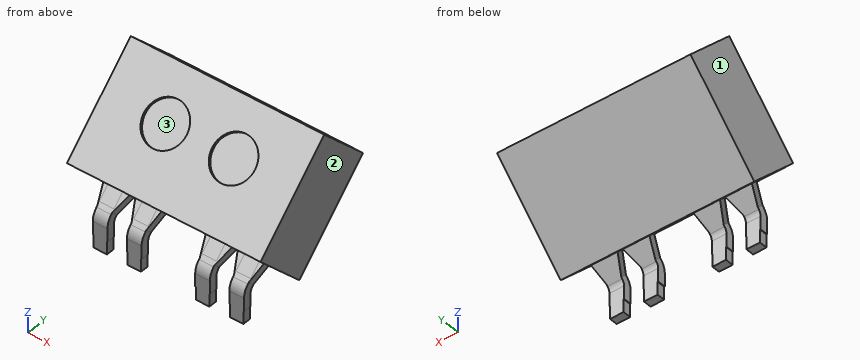
```python
from build123d import *

# Parameters (mm, degrees)
ESQUISSE2_W          = 7.2
ESQUISSE2_H          = 2.5
BOITIER_DEPTH        = 4.1
FENETRECAPTEUR_START = -1.45
ESQUISSE4_R          = 0.8
FENETRECAPTEUR_DEPTH = 0.1
PATTES_DEPTH         = 0.15
PLIAGE_START         = -5
PLIAGE_1_OUTLINE_W   = 7.2
PLIAGE_1_OUTLINE_H   = 4.1
PLIAGE_1_DEPTH       = 4.301040764
PLIAGE_START_2       = -0.698959236
PLIAGE_1_2_OUTLINE_R = 0.8
PLIAGE_1_2_DEPTH     = 0.1
PLIAGE_START_3       = -0.598959236
PLIAGE_1_3_OUTLINE_W = 7.2
PLIAGE_1_3_OUTLINE_H = 4.1
PLIAGE_1_3_DEPTH     = 2.4
PLIAGE_1_4_OUTLINE_W = 7.2
PLIAGE_1_4_OUTLINE_H = 4.1
PLIAGE_1_4_OUTLINE_R = 0.8
PLIAGE_1_4_DEPTH     = 0.1
PLIAGE_START_4       = -3.6
PLIAGE_1_5_DEPTH     = 7.2
PLIAGE_START_5       = -2.813242849
PLIAGE_1_6_DEPTH     = 0.546485698
PLIAGE_START_6       = -1.543242849
PLIAGE_1_7_DEPTH     = 0.546485698
PLIAGE_START_7       = 0.996757151
PLIAGE_1_8_DEPTH     = 0.546485698
PLIAGE_START_8       = 2.266757151
PLIAGE_1_9_DEPTH     = 0.546485698
PLIAGE_START_9       = 0.601040763
PLIAGE_1_10_DEPTH    = 0.300000001


with BuildPart() as part:
    # Esquisse2 → Boitier (new body)
    with BuildSketch(Plane.XY):
        with Locations((0, -0.2)):
            Rectangle(ESQUISSE2_W, ESQUISSE2_H)
    extrude(amount=BOITIER_DEPTH)

    # Esquisse4 → FenetreCapteur (cut)
    with BuildSketch(Plane(origin=(0, 0, 0), x_dir=(1, 0, 0), z_dir=(0, 1, 0)).offset(FENETRECAPTEUR_START)):
        with Locations(Location((-1.27, -2.3, 0), (0, 0, 180))):
            Circle(ESQUISSE4_R)
        with Locations(Location((1.27, -2.3, 0), (0, 0, 180))):
            Circle(ESQUISSE4_R)
    extrude(amount=FENETRECAPTEUR_DEPTH, mode=Mode.SUBTRACT)

    # Esquisse5 → Pattes (add, symmetric)
    with BuildSketch(Plane(origin=(0, 0, 0), x_dir=(1, 0, 0), z_dir=(0, 1, 0))):
        Polygon((2.791437744, 2.2), (2.283797649, 2.2), (2.283797649, 1.724539267), (2.266757151, 1.724539267), (2.266757151, 0.7), (2.002499851, 0), (2.991852509, 0), (2.813242849, 0.7), (2.813242849, 1.724539267), (2.791437744, 1.724539267), align=None)
        Polygon((1.526202351, 2.2), (1.018562256, 2.2), (1.018562256, 1.724539267), (0.996757151, 1.724539267), (0.996757151, 0.7), (0.818147491, 0), (1.807500149, 0), (1.543242849, 0.7), (1.543242849, 1.724539267), (1.526202351, 1.724539267), align=None)
        Polygon((-1.018562256, 2.2), (-1.526202351, 2.2), (-1.526202351, 1.724539267), (-1.543242849, 1.724539267), (-1.543242849, 0.7), (-1.807500149, 0), (-0.818147491, 0), (-0.996757151, 0.7), (-0.996757151, 1.724539267), (-1.018562256, 1.724539267), align=None)
        Polygon((-2.283797649, 2.2), (-2.791437744, 2.2), (-2.791437744, 1.724539267), (-2.813242849, 1.724539267), (-2.813242849, 0.7), (-2.991852509, 0), (-2.002499851, 0), (-2.266757151, 0.7), (-2.266757151, 1.724539267), (-2.283797649, 1.724539267), align=None)
    extrude(amount=PATTES_DEPTH, both=True)

    # Pliage 1: read off the stored shape, not the designer's step
    # Pliage 1 outline → Pliage 1 (cut)
    with BuildSketch(Plane(origin=(0, 0, 0), x_dir=(1, 0, 0), z_dir=(0, 0.707106781186546, -0.707106781186549)).offset(PLIAGE_START)):
        with Locations((0, -2.236827202)):
            Rectangle(PLIAGE_1_OUTLINE_W, PLIAGE_1_OUTLINE_H)
    extrude(amount=PLIAGE_1_DEPTH, mode=Mode.SUBTRACT)

    # Pliage 1 2 outline → Pliage 1 2 (cut)
    with BuildSketch(Plane(origin=(0, 0, 0), x_dir=(1, 0, 0), z_dir=(0, 0.707106781186546, -0.707106781186549)).offset(PLIAGE_START_2)):
        with Locations((-1.27, -2.486827202)):
            Circle(PLIAGE_1_2_OUTLINE_R)
        with Locations((1.27, -2.486827202)):
            Circle(PLIAGE_1_2_OUTLINE_R)
    extrude(amount=PLIAGE_1_2_DEPTH, mode=Mode.SUBTRACT)

    # Pliage 1 3 outline → Pliage 1 3 (add)
    with BuildSketch(Plane(origin=(0, 0, 0), x_dir=(1, 0, 0), z_dir=(0, 0.707106781186546, -0.707106781186549)).offset(PLIAGE_START_3)):
        with Locations((0, -2.236827202)):
            Rectangle(PLIAGE_1_3_OUTLINE_W, PLIAGE_1_3_OUTLINE_H)
    extrude(amount=PLIAGE_1_3_DEPTH)

    # Pliage 1 4 outline → Pliage 1 4 (add)
    with BuildSketch(Plane(origin=(0, 0, 0), x_dir=(1, 0, 0), z_dir=(0, 0.707106781186546, -0.707106781186549)).offset(PLIAGE_START_2)):
        with Locations((0, -2.236827202)):
            Rectangle(PLIAGE_1_4_OUTLINE_W, PLIAGE_1_4_OUTLINE_H)
        with Locations((-1.27, -2.486827202)):
            Circle(PLIAGE_1_4_OUTLINE_R, mode=Mode.SUBTRACT)
        with Locations((1.27, -2.486827202)):
            Circle(PLIAGE_1_4_OUTLINE_R, mode=Mode.SUBTRACT)
    extrude(amount=PLIAGE_1_4_DEPTH)

    # Pliage 1 5 outline → Pliage 1 5 (cut)
    with BuildSketch(Plane.YZ.offset(PLIAGE_START_4)):
        with BuildLine():
            Line((0.021781873, -0.828218127), (0.15, -0.7))
            Line((0.15, -0.7), (0.15, 0))
            Line((0.15, 0), (0.264213563, 0))
            Line((0.264213563, 0), (-1.35, 1.614213563))
            Line((-1.35, 1.614213563), (-1.45, 1.714213563))
            Line((-1.45, 1.714213563), (-1.45, 0))
            Line((-1.45, 0), (-0.15, 0))
            Line((-0.15, 0), (-0.15, -1.242936254))
            ThreePointArc((-0.15, -1.242936254), (-0.105355346, -1.018492421), (0.021781873, -0.828218127))
        make_face()
    extrude(amount=PLIAGE_1_5_DEPTH, mode=Mode.SUBTRACT)

    # Pliage 1 6 outline → Pliage 1 6 (add)
    with BuildSketch(Plane.YZ.offset(PLIAGE_START_5)):
        with BuildLine():
            Line((0.769238816, -0.505025253), (0.557106781, -0.292893218))
            Line((0.557106781, -0.292893218), (0.15, -0.7))
            Line((0.15, -0.7), (0.15, -1.242936254))
            ThreePointArc((0.15, -1.242936254), (0.171808514, -1.133297451), (0.233913907, -1.040350162))
            Line((0.233913907, -1.040350162), (0.769238816, -0.505025253))
        make_face()
    extrude(amount=PLIAGE_1_6_DEPTH)

    # Pliage 1 7 outline → Pliage 1 7 (add)
    with BuildSketch(Plane.YZ.offset(PLIAGE_START_6)):
        with BuildLine():
            Line((0.769238816, -0.505025253), (0.557106781, -0.292893218))
            Line((0.557106781, -0.292893218), (0.15, -0.7))
            Line((0.15, -0.7), (0.15, -1.242936254))
            ThreePointArc((0.15, -1.242936254), (0.171808514, -1.133297451), (0.233913907, -1.040350162))
            Line((0.233913907, -1.040350162), (0.769238816, -0.505025253))
        make_face()
    extrude(amount=PLIAGE_1_7_DEPTH)

    # Pliage 1 8 outline → Pliage 1 8 (add)
    with BuildSketch(Plane.YZ.offset(PLIAGE_START_7)):
        with BuildLine():
            Line((0.769238816, -0.505025253), (0.557106781, -0.292893218))
            Line((0.557106781, -0.292893218), (0.15, -0.7))
            Line((0.15, -0.7), (0.15, -1.242936254))
            ThreePointArc((0.15, -1.242936254), (0.171808514, -1.133297451), (0.233913907, -1.040350162))
            Line((0.233913907, -1.040350162), (0.769238816, -0.505025253))
        make_face()
    extrude(amount=PLIAGE_1_8_DEPTH)

    # Pliage 1 9 outline → Pliage 1 9 (add)
    with BuildSketch(Plane.YZ.offset(PLIAGE_START_8)):
        with BuildLine():
            Line((0.769238816, -0.505025253), (0.557106781, -0.292893218))
            Line((0.557106781, -0.292893218), (0.15, -0.7))
            Line((0.15, -0.7), (0.15, -1.242936254))
            ThreePointArc((0.15, -1.242936254), (0.171808514, -1.133297451), (0.233913907, -1.040350162))
            Line((0.233913907, -1.040350162), (0.769238816, -0.505025253))
        make_face()
    extrude(amount=PLIAGE_1_9_DEPTH)

    # Pliage 1 10 outline → Pliage 1 10 (add)
    with BuildSketch(Plane(origin=(0, 0, 0), x_dir=(1, 0, 0), z_dir=(0, 0.707106781186546, -0.707106781186549)).offset(PLIAGE_START_9)):
        Polygon((2.813242849, 0.513172798), (2.813242849, -0.186827202), (2.991852509, -0.186827202), align=None)
        Polygon((-2.991852509, -0.186827202), (-2.813242849, -0.186827202), (-2.813242849, 0.513172798), align=None)
        Polygon((-2.266757151, -0.186827202), (-2.002499851, -0.186827202), (-2.266757151, 0.513172798), align=None)
        Polygon((-1.807500149, -0.186827202), (-1.543242849, -0.186827202), (-1.543242849, 0.513172798), align=None)
        Polygon((-0.996757151, -0.186827202), (-0.818147491, -0.186827202), (-0.996757151, 0.513172798), align=None)
        Polygon((0.818147491, -0.186827202), (0.996757151, -0.186827202), (0.996757151, 0.513172798), align=None)
        Polygon((1.543242849, -0.186827202), (1.807500149, -0.186827202), (1.543242849, 0.513172798), align=None)
        Polygon((2.266757151, 0.513172798), (2.002499851, -0.186827202), (2.266757151, -0.186827202), align=None)
    extrude(amount=PLIAGE_1_10_DEPTH)


solid = part.part
```
Design review of the part built by this model. Coordinates are the model's own, in mm. Face numbers are marked on the shaded views. Coordinates: 2 decimals unless noted, no trailing zeros. Write each loop counter-clockwise with the first axis right and the second up, starting at its lowest first coordinate (ties: lowest second). Pieces come first, ordered by that corner, then holes.
1) Add section A-A (z = -1.55). Write out the cut boundary in (x, y), plus the area to 3 significant figures.
2) Mouldability with a two-part tool opening along X and no side actions: class the marked faces 1, 2 and 3 as +X half, -X half, draft (parallel to the pull), parting line (faces both ways), or undercut.
3) Insertion check: pin 1 (0.5 mm diameter, centred on y = 0, z = -1, fed in from +X); pin 2 (3 mm diameter, centred on x = -1.5, z = 1.5, fed in from +Y); pin 3 (1.5 mm diameter, centred on x = 0, y = 0.5, fed in from +Z); pin 4 (0.5 mm diameter, centred on y = 0, z = -1, fed in from -X). Each pin has a flat end and moves straight along its axis. Give the tip position at first contact, or say it passes through.
4) Add section C-C (x = 2.5). Write out the cut boundary in (y, z).
5) Add section D-D (y = 2.1). Write out the cut boundary in (x, z), plus the area to 3 significant figures.
6) Add section B-B (y = 0.45). Write out the cut boundary in (x, z), plus the area to 4 significant figures.
7) To check wall thickness, follow L1, parallel to Z at x = 0, y = 0; L2, parallel to Y at x = 0, z = 1.25; L3, parallel to Z at x = -1.5, y = -0.2. State the ranges of each line that lie inside material, in increasing order.
Check result:
1. outline: (-2.81, -0.15) - (-2.27, -0.15) - (-2.27, 0.15) - (-2.81, 0.15) - close; (-1.54, -0.15) - (-1, -0.15) - (-1, 0.15) - (-1.54, 0.15) - close; (1, -0.15) - (1.54, -0.15) - (1.54, 0.15) - (1, 0.15) - close; (2.27, -0.15) - (2.81, -0.15) - (2.81, 0.15) - (2.27, 0.15) - close
1. area: 0.656 mm2
2. face 1: -X half
2. face 2: +X half
2. face 3: undercut
3. pin 1: stops at x = 2.83
3. pin 2: stops at y = 4.3
3. pin 3: stops at z = 2.24
3. pin 4: stops at x = -2.83
4. outline: (-0.36, 0.63) - (0.56, -0.29) - (0.02, -0.83) arc R0.59 ccw to (-0.15, -1.24) - (-0.15, -2.2) - (0.15, -2.2) - (0.15, -1.24) arc R0.29 cw to (0.23, -1.04) - (0.77, -0.51) - (1.41, -1.14) - (4.3, 1.76) - (2.54, 3.53) - close
5. outline: (-3.6, -0.45) - (3.6, -0.45) - (3.6, 3.09) - (-3.6, 3.09) - close
5. area: 25.5 mm2
6. outline: (-3.6, -0.19) - (3.6, -0.19) - (3.6, 1.44) - (-3.6, 1.44) - close; (-2.95, -0.4) - (-2.88, -0.82) - (-2.17, -0.82) - (-2.06, -0.4) - close; (-1.75, -0.4) - (-1.64, -0.82) - (-0.93, -0.82) - (-0.86, -0.4) - close; (0.86, -0.4) - (0.93, -0.82) - (1.64, -0.82) - (1.75, -0.4) - close; (2.06, -0.4) - (2.17, -0.82) - (2.88, -0.82) - (2.95, -0.4) - close
6. area: 13.05 mm2
7. L1: z = 0.26 to 0.99
7. L2: y = 0.26 to 3.8
7. L3: z = 0.46 to 0.79
